```python
from build123d import *

# Parameters (mm, degrees)
BOSS_EXTRU_1_DEPTH = 5
ESQUISSE14_W       = 30.8
ESQUISSE14_H       = 2.5
BOSS_EXTRU_3_DEPTH = 10
BOSS_EXTRU_5_DEPTH = 35


with BuildPart() as part:
    # Base → Boss.-Extru.1 (new, symmetric)
    with BuildSketch(Plane(origin=(0, 0, 0), x_dir=(1, 0, 0), z_dir=(0, 1, 0))):
        Polygon((-3.85, -2.4), (-3.85, 2.4), (-10.1, 2.4), (-10.1, 10.1), (-2.4, 10.1), (-2.4, 3.85), (2.4, 3.85), (2.4, 10.1), (10.1, 10.1), (10.1, 2.4), (3.85, 2.4), (3.85, -2.4), (10.1, -2.4), (10.1, -6.25), (15.4, -6.25), (15.4, 15.4), (-15.4, 15.4), (-15.4, -6.25), (-10.1, -6.25), (-10.1, -2.4), align=None)
    extrude(amount=BOSS_EXTRU_1_DEPTH, both=True)

    # Esquisse14 → Boss.-Extru.3 (add)
    with BuildSketch(Plane.XZ.offset(5)):
        with Locations((0, -16.65)):
            Rectangle(ESQUISSE14_W, ESQUISSE14_H)
    extrude(amount=-BOSS_EXTRU_3_DEPTH)

    # Esquisse16 → Boss.-Extru.5 (add)
    with BuildSketch(Plane(origin=(0, 0, -17.9), x_dir=(-1, 0, 0), z_dir=(0, 0, -1))):
        Polygon((31.226270189, 20.920127019), (33.726270189, 16.59), (-9.575, -8.41), (-12.075, -4.079872981), align=None)
    extrude(amount=BOSS_EXTRU_5_DEPTH)


solid = part.part
```
The model under review builds one solid part; all positions refer to its coordinate system, in mm. A direction names the side the tool comes from. Round coordinates to 2 decimals unless told otherwise and drop trailing zeros. Write each loop counter-clockwise with the first axis right and the second up, starting at its lowest first coordinate (ties: lowest second). Pieces come first, ordered by that corner, then holes. Notation, with made-up numbers: M 61.25,-31.75 L 112.25,-31.75 A24 ccw 112.25,-14.75 Z; hole C 43.5,76.5 d7. An arc over 180 degrees is marked long. Use CSV: the item, a comma, the result in double quotes. Start each with the question number.
(1) We need section A-A, the plane z = 0. State the section outline as (x, y) points, then the cut area to 3 significant figures.
(2) We need section C-C, the plane x = 1. State the section outline as (y, z) points.
(3) For line 1 along X through (y, z) = (-2.75, -8); line 2 along Z through (x, y) = (-6, 3.5); line 3 along Z through (x, y) = (6, -0.25), list the stretches that pass through material, from the lowest coordinate up.
(4) We need section B-B, the plane x = -5.5. State the section outline as (y, z) points.
(5) Clearance check with flat-ended pins moving along their axes: P1, Ø8, axis at x = -9.5, y = 2, coming from the -Z side; P2, Ø6, axis at x = -12.5, z = -27.5, coming from the -Y side; P3, Ø1.9, axis at x = -7.5, y = -1, coming from the +Z side; P4, Ø1.4, axis at y = 1, z = 1, coming from the -X side. State where each tip first meets the part, or that it passes through.
(6) The part is to be moulded in two halves that separate along X. For faces 4 (the face through (-10.1, 0, -6)), 5 (the face through (15.4, 0, -6)), 6 (the face through (-15.4, 0, -6)), say which applies: +X half, -X half, draft (parallel to the pull), parting line (faces both ways), or undercut.
(7) We need section D-D, the plane y = -2.5. State the section outline as (x, z) points, then the cut area to 3 significant figures.
(8) Tool access review of faces 1 (the face through (-9.273, 8.245, -35.155)), 2 (the face through (-10.1, 0, 4)), 3 (the face through (-12.379, 4.265, -35.155)): name each direction out of +Z, -Z, +X, -X, +Y, -Y from which nothing blocks a thin tool from reaching the whole face with its end or side.
Findings:
1,outline,"M -15.4,-5 L -3.85,-5 L -3.85,5 L -15.4,5 Z; M 3.85,-5 L 15.4,-5 L 15.4,5 L 3.85,5 Z"
1,area,"231 mm^2"
2,outline,"M -5,-17.9 L -3.46,-17.9 L -3.46,-52.9 L 2.31,-52.9 L 2.31,-17.9 L 5,-17.9 L 5,-3.85 L -5,-3.85 Z"
3,line 1,"-15.4 to -10.1, -2.4 to 2.4, 10.1 to 15.4"
3,line 2,"-52.9 to -10.1, -2.4 to 2.4"
3,line 3,"-17.9 to -10.1, -2.4 to 2.4"
4,outline,"M -5,-17.9 L 0.29,-17.9 L 0.29,-52.9 L 6.07,-52.9 L 6.07,-17.9 L 5,-17.9 L 5,-10.1 L -5,-10.1 Z; M -5,-2.4 L 5,-2.4 L 5,2.4 L -5,2.4 Z"
5,P1,"z = -52.9"
5,P2,"y = 2.6"
5,P3,"z = 2.4"
5,P4,"x = -15.4"
6,face 4,"undercut"
6,face 5,"+X half"
6,face 6,"-X half"
7,outline,"M -15.4,-17.9 L -0.66,-17.9 L -0.66,-52.9 L 9.34,-52.9 L 9.34,-17.9 L 15.4,-17.9 L 15.4,6.25 L 10.1,6.25 L 10.1,2.4 L 3.85,2.4 L 3.85,-2.4 L 10.1,-2.4 L 10.1,-10.1 L 2.4,-10.1 L 2.4,-3.85 L -2.4,-3.85 L -2.4,-10.1 L -10.1,-10.1 L -10.1,-2.4 L -3.85,-2.4 L -3.85,2.4 L -10.1,2.4 L -10.1,6.25 L -15.4,6.25 Z"
7,area,"854 mm^2"
8,face 1,"-Z, +X, +Y"
8,face 2,"+Z, +Y, -Y"
8,face 3,"-Z, -X, -Y"
